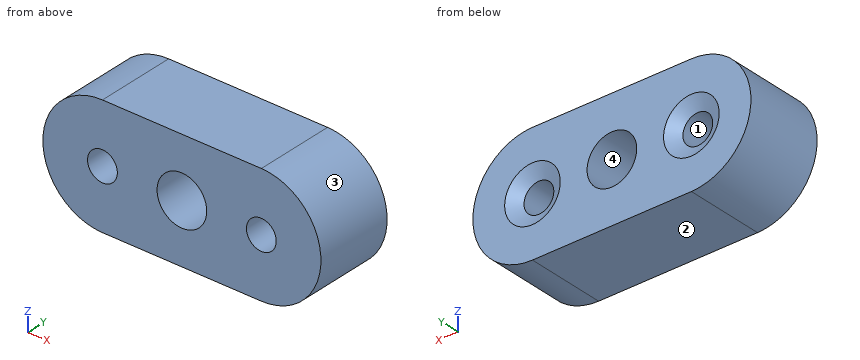
from build123d import *

# Parameters (mm, degrees)
SKETCH1_R           = 3.96875
BOSS_EXTRUDE1_DEPTH = 12.7


with BuildPart() as part:
    # Sketch1 → Boss-Extrude1 (new body)
    with BuildSketch(Plane(origin=(0, 0, 0), x_dir=(1, 0, 0), z_dir=(0, 1, 0))):
        with BuildLine():
            Line((-12.7, 9.525), (12.7, 9.525))
            ThreePointArc((12.7, 9.525), (22.225, 0), (12.7, -9.525))
            Line((12.7, -9.525), (-12.7, -9.525))
            ThreePointArc((-12.7, -9.525), (-22.225, 0), (-12.7, 9.525))
        make_face()
        Circle(SKETCH1_R, mode=Mode.SUBTRACT)
    extrude(amount=BOSS_EXTRUDE1_DEPTH)

    # Sketch2 → Cut-Revolve1 (revolve, cut)
    with BuildSketch(Plane.XY):
        Polygon((-12.7, 12.7), (-17.145, 12.7), (-15.08125, 11.459973897), (-15.08125, 0), (-12.7, 0), align=None)
    cut_revolve1 = revolve(axis=Axis((-12.7, 0, 0), (0, 1, 0)), mode=Mode.SUBTRACT)

    # Mirror1: Cut-Revolve1 across plane
    add(cut_revolve1.mirror(Plane(origin=(0, 0, 0), x_dir=(0, 0, 1), z_dir=(1, 0, 0))), mode=Mode.SUBTRACT)


solid = part.part
Model file for the job. Use its own axes, mm. Face numbers are marked on the shaded views. Round coordinates to 2 decimals unless told otherwise and drop trailing zeros. Loops run counter-clockwise (first coordinate to the right, second up) from the corner with the lowest first, then second, coordinate; pieces in that order, holes last. Notation, with made-up numbers: M 34.25,-16 L 71.25,-16 A22 cw 71.25,16 Z; hole C -36,-22 d4. An arc over 180 degrees is marked long. One line per question, with ' | ' between items.
1) Drill centre lines: line 1 along Z through (x, y) = (12.7, 7) (3 decimals); line 2 along Z through (x, y) = (0, 7.5) (3 decimals); line 3 along X through (y, z) = (10.25, -1.25). Where is each one in solid material? Low to high.
Solved:
line 1: z = -9.525 to -2.381, 2.381 to 9.525 | line 2: z = -9.525 to -3.969, 3.969 to 9.525 | line 3: x = -22.14 to -14.73, -10.67 to -3.77, 3.77 to 10.67, 14.73 to 22.14
2) Mould opens along X. For the marked faces 1, 2, 3 and 4 say: +X half, -X half, draft (parallel to the pull), parting line (faces both ways), or undercut.
Solved:
face 1: undercut | face 2: draft | face 3: +X half | face 4: undercut
3) Flat gauge pins, fed straight in: pin 1 (7.5 mm diameter, centred on x = 12.7, z = 0, fed in from +Y); pin 2 (4 mm diameter, centred on x = -12.7, z = 0, fed in from -Y). Where does each tip first touch, or does it go through?
Solved:
pin 1: stops at y = 12.28 | pin 2: passes through
4) Band-saw the part on D-D (z = 6.75). Give the cut face in (x, y), then the cut area to 3 significant figures.
Solved:
outline: M -19.42,0 L 19.42,0 L 19.42,12.7 L -19.42,12.7 Z | area: 493 mm²
5) Band-saw the part on B-B (x = 0). Give the cut face in (y, z) (3 decimals), then the cut area to 3 significant figures.
Solved:
outline: M 0,-9.525 L 12.7,-9.525 L 12.7,-3.969 L 0,-3.969 Z; M 0,3.969 L 12.7,3.969 L 12.7,9.525 L 0,9.525 Z | area: 141 mm²
6) Band-saw the part on A-A (z = 0). Give the cut face in (x, y) (3 decimals), then the cut area to 3 significant figures.
Solved:
outline: M -22.225,0 L -15.081,0 L -15.081,11.46 L -17.145,12.7 L -22.225,12.7 Z; M -10.319,0 L -3.969,0 L -3.969,12.7 L -8.255,12.7 L -10.319,11.46 Z; M 3.969,0 L 10.319,0 L 10.319,11.46 L 8.255,12.7 L 3.969,12.7 Z; M 15.081,0 L 22.225,0 L 22.225,12.7 L 17.145,12.7 L 15.081,11.46 Z | area: 338 mm²
7) Band-saw the part on C-C (y = 8). Give the number of separate pieces and of enclosed holes in the cut face, then the cut area to 3 significant figures.
Solved:
separate pieces: 1 | enclosed holes: 3 | area: 684 mm²
